from build123d import *

# Parameters (mm, degrees)
F0_W     = 67
F0_H     = 5
F1_DEPTH = 10.2
F2_W     = 67
F2_H     = 25
F2_H_2   = 5
F3_DEPTH = 5
F4_SIZE  = 4.99999
F5_W     = 67
F5_H     = 5
F5_H_2   = 25
F6_DEPTH = 5
F7_SIZE  = 4.99999


# Not quite as in the source:
# - a fillet or chamfer is up to 0.001 mm smaller than in the source, because OpenCascade refuses the exact size


with BuildPart() as f1:
    # F0 (on Top) → F1 (new body)
    with BuildSketch(Plane.XY):
        Rectangle(F0_W, F0_H)
    extrude(amount=F1_DEPTH)

    # F2 (on face) → F3 (join)
    with BuildSketch(Plane.XY.offset(10.2)):
        with Locations((0, -15)):
            Rectangle(F2_W, F2_H)
        Rectangle(F2_W, F2_H_2)
    extrude(amount=F3_DEPTH)

    # F4 (size 5 in the source; OpenCascade refuses exactly that, so slightly less here)
    f4_edges = [f1.edges().sort_by_distance(p)[0] for p in [
        (0, -27.5, 15.2),
    ]]
    chamfer(f4_edges, length=F4_SIZE)

    # F5 (on face) → F6 (join)
    with BuildSketch(Plane(origin=(0, 0, 0), x_dir=(1, 0, 0), z_dir=(0, 0, -1))):
        Rectangle(F5_W, F5_H)
        with Locations((0, 15)):
            Rectangle(F5_W, F5_H_2)
    extrude(amount=F6_DEPTH)

    # F7 (size 5 in the source; OpenCascade refuses exactly that, so slightly less here)
    f7_edges = [f1.edges().sort_by_distance(p)[0] for p in [
        (0, -27.5, -5),
    ]]
    chamfer(f7_edges, length=F7_SIZE)


solid = f1.part
Verification items for the finished model (mm, model axes). A direction names the side the tool comes from. Give positions to 0.01 mm unless a question says otherwise; leave off trailing zeros. Write each loop counter-clockwise with the first axis right and the second up, starting at its lowest first coordinate (ties: lowest second). Pieces come first, ordered by that corner, then holes. Notation, with made-up numbers: M 35,-29.75 L 87,-29.75 A7 ccw 87,-23.75 Z; hole C -30.75,-10.75 d7. An arc over 180 degrees is marked long. Write item = value, one per line.
(1) Sectioned sample at A-A (y = -3.5). Record the cut outline in (x, z).
Found:
outline = M -33.5,-5 L 33.5,-5 L 33.5,0 L -33.5,0 Z; M -33.5,10.2 L 33.5,10.2 L 33.5,15.2 L -33.5,15.2 Z
(2) Sectioned sample at C-C (y = -26). Record the cut outline in (x, z).
Found:
outline = M -33.5,-1.5 L 33.5,-1.5 L 33.5,0 L -33.5,0 Z; M -33.5,10.2 L 33.5,10.2 L 33.5,11.7 L -33.5,11.7 Z
(3) Draft check along Z on faces 3 (the face through (-0.5, -25, -2.5)), 4 (the face through (0, -15, 0)), 5 (the face through (-0.5, -25, 12.7)), 6 (the face through (33.5, -9, 12)). Enter one of: released by +Z, released by -Z, zero draft, split by the parting line, or undercut.
Found:
face_3 = released by -Z
face_4 = undercut
face_5 = released by +Z
face_6 = zero draft
(4) Go/stop test with flat-tipped pins: pin 1 Ø1 at (x, z) = (2, 9.5) entering from -Y; pin 2 Ø8 at (x, z) = (-8.5, 7.5) entering from -Y. Record where each tip stops, or that it passes through.
Found:
pin_1 = -2.5
pin_2 = -27.5
(5) Sectioned sample at D-D (z = 2.75). Record the cut outline in (x, y), then the cut area to 3 significant figures.
Found:
outline = M -33.5,-2.5 L 33.5,-2.5 L 33.5,2.5 L -33.5,2.5 Z
area = 335 mm2
(6) Material ranges on line 1 (Z direction, x = -7.5, y = -16.5); line 2 (Z direction, x = 28, y = -26); line 3 (Y direction, x = -24, z = 4), recorded low to high.
Found:
line_1 = -5 to 0, 10.2 to 15.2
line_2 = -1.5 to 0, 10.2 to 11.7
line_3 = -2.5 to 2.5
(7) Access from +Z, -Z, +X, -X, +Y, -Y to the whole of each face (thin tool, end or side, straight path). Record for faces 1 (the face through (0, -10, -5)), 2 (the face through (0, -15, 10.2)).
Found:
face_1 = -Z, +X, -X, +Y, -Y
face_2 = +X, -X, -Y
